Geometry: final body of the model. Coordinates: model frame, mm. Face numbers are marked on the shaded views. Give positions to 0.01 mm unless a question says otherwise; leave off trailing zeros. Write each loop counter-clockwise with the first axis right and the second up, starting at its lowest first coordinate (ties: lowest second). Pieces come first, ordered by that corner, then holes.
from build123d import *

# Parameters (mm, degrees)
SKETCH_1_R          = 2
EXTRUDE_1_DEPTH     = 2
SKETCH_3_W          = 3
SKETCH_3_H          = 14.5
CUT_EXTRUDE_1_DEPTH = 1
SKETCH_4_W          = 42
SKETCH_4_H          = 17
SKETCH_4_W_2        = 40
SKETCH_4_H_2        = 15
EXTRUDE_2_DEPTH     = 1
SKETCH_6_W          = 5.5
SKETCH_6_H          = 15
SKETCH_6_W_2        = 3.5
EXTRUDE_4_DEPTH     = 1
SKETCH_7_W          = 42
SKETCH_7_H          = 17
SKETCH_7_W_2        = 31
SKETCH_7_H_2        = 15
EXTRUDE_5_DEPTH     = 1


with BuildPart() as part:
    # 草图1 → 凸台-拉伸1 (new body)
    with BuildSketch(Plane.XY):
        Polygon((-30, 8.5), (-30, -8.5), (12, -8.5), (12, 0), (12, 8.5), align=None)
        Circle(SKETCH_1_R, mode=Mode.SUBTRACT)
    extrude(amount=EXTRUDE_1_DEPTH)

    # 草图3 → 切除-拉伸1 (cut)
    with BuildSketch(Plane.XY.offset(2)):
        with Locations((-22, 0)):
            Rectangle(SKETCH_3_W, SKETCH_3_H)
        Polygon((7.5, 7.25), (5, 7.25), (5, -7.25), (7.5, -7.25), (7.5, 0), align=None)
    extrude(amount=-CUT_EXTRUDE_1_DEPTH, mode=Mode.SUBTRACT)

    # 草图4 → 凸台-拉伸2 (add)
    with BuildSketch(Plane.XY.offset(2)):
        with Locations((-9, 0)):
            Rectangle(SKETCH_4_W, SKETCH_4_H)
        with Locations((-9, 0)):
            Rectangle(SKETCH_4_W_2, SKETCH_4_H_2, mode=Mode.SUBTRACT)
    extrude(amount=EXTRUDE_2_DEPTH)

    # 草图6 → 凸台-拉伸4 (add)
    with BuildSketch(Plane.XY.offset(2)):
        with Locations((-26.25, 0)):
            Rectangle(SKETCH_6_W, SKETCH_6_H)
        with Locations((9.25, 0)):
            Rectangle(SKETCH_6_W_2, SKETCH_6_H)
    extrude(amount=EXTRUDE_4_DEPTH)

    # 草图7 → 凸台-拉伸5 (add)
    with BuildSketch(Plane.XY.offset(3)):
        with Locations((-9, 0)):
            Rectangle(SKETCH_7_W, SKETCH_7_H)
        with Locations((-8, 0)):
            Rectangle(SKETCH_7_W_2, SKETCH_7_H_2, mode=Mode.SUBTRACT)
    extrude(amount=EXTRUDE_5_DEPTH)


solid = part.part
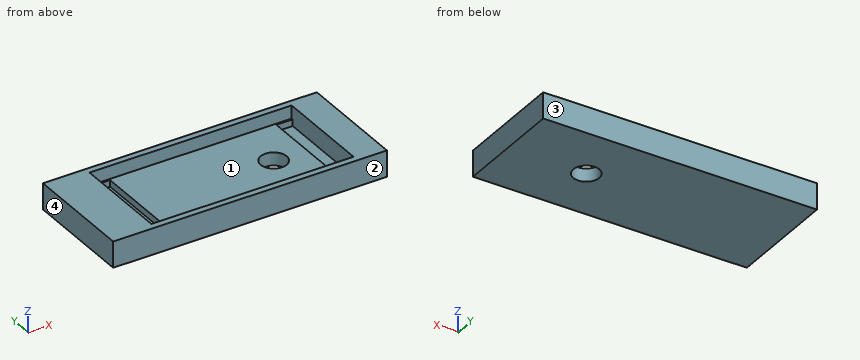
Q1. Section A-A on x = 0. Output: boundary loops of the cut face in (y, z), plus the area to 3 significant figures.
Filled sheet:
outline: (-8.5, 0) - (-2, 0) - (-2, 2) - (-7.5, 2) - (-7.5, 4) - (-8.5, 4) - close; (2, 0) - (8.5, 0) - (8.5, 4) - (7.5, 4) - (7.5, 2) - (2, 2) - close
area: 30.0 mm2
Q2. Pull-direction query (Y, two-part tool) for the marked faces 1, 2, 3 and 4; classes: released by +Y, released by -Y, zero draft, split by the parting line, or undercut.
Filled sheet:
face 1: undercut
face 2: released by -Y
face 3: released by +Y
face 4: zero draft
Q3. Section C-C on z = 3.3. Output: boundary loops of the cut face in (x, y).
Filled sheet:
outline: (-30, -8.5) - (12, -8.5) - (12, 8.5) - (-30, 8.5) - close; hole (-23.5, -7.5) - (7.5, -7.5) - (7.5, 7.5) - (-23.5, 7.5) - close
Q4. Section B-B on y = 0. Output: boundary loops of the cut face in (x, z), plus the area to 3 significant figures.
Filled sheet:
outline: (-30, 0) - (-2, 0) - (-2, 2) - (-20.5, 2) - (-20.5, 1) - (-23.5, 1) - (-23.5, 4) - (-30, 4) - close; (2, 0) - (12, 0) - (12, 4) - (7.5, 4) - (7.5, 1) - (5, 1) - (5, 2) - (2, 2) - close
area: 92.5 mm2
Q5. Ray query, line 1 along X through (y, z) = (5.75, 1.65); line 2 along Y through (x, z) = (0, 0.95); line 3 along X through (y, z) = (-6.75, 3.55). Return the intervals inside material, ascending.
Filled sheet:
line 1: x = -30 to -23.5, -20.5 to 5, 7.5 to 12
line 2: y = -8.5 to -2, 2 to 8.5
line 3: x = -30 to -23.5, 7.5 to 12
Q6. Pin query (flat end, axial travel): P1, Ø4.5, axis at x = -11.5, y = 2, coming from the +Z side; P2, Ø1.5, axis at x = -22, y = 1, coming from the +Z side; P3, Ø2.5, axis at x = 0, y = 0, coming from the +Z side. Return the tip coordinate at first contact, or that it passes through.
Filled sheet:
P1: stops at z = 2
P2: stops at z = 1
P3: passes through
Q7. Section D-D on z = 1.55. Output: boundary loops of the cut face in (x, y), plus the area to 3 significant figures.
Filled sheet:
outline: (-30, -8.5) - (12, -8.5) - (12, 8.5) - (-30, 8.5) - close; hole (-23.5, -7.25) - (-20.5, -7.25) - (-20.5, 7.25) - (-23.5, 7.25) - close; hole circle Ø4 at (0, 0); hole (5, -7.25) - (7.5, -7.25) - (7.5, 7.25) - (5, 7.25) - close
area: 622 mm2
